The listing builds one solid part. Answer for the finished solid, in the listing's coordinates (mm). A direction names the side the tool comes from. Coordinates: 2 decimals unless noted, no trailing zeros. Order: outer loops, then holes, each group sorted by start corner. A loop starts at its lowest first (then second) coordinate and runs counter-clockwise, first axis right, second up. Notation, with made-up numbers: M -34.5,-28.75 L 22.5,-28.75 A21 cw 22.5,-6.75 Z; hole C -33.5,34.5 d7. An arc over 180 degrees is marked long. One line per item, written item: value. Start each with the question number.
Q1. This flat-tipped pin is pushed along its axis until it touches: pin 1 Ø2.5 at (y, z) = (-2, 4) entering from +X. Where does it stop, or does it pass through?
Q2. For faces 1 (the cylindrical face through (3, 4, 1)), 2 (the flat face through (-3, 0, 2.5)), determine the directions among +Z, -Z, +X, -X, +Y, -Y from which every point of the face is accessible in a straight line to the end or side of a thin tool.
Q3. The part is cut by section D-D on z = 8.25. Give the vertices of the cut face in (x, y), then the cut area to 3 significant figures.
Q4. The part is cut by section C-C on z = 5. Give the vertices of the cut face in (x, y).
Q5. The part is cut by section A-A on y = 0. Give the vertices of the cut face in (x, z), then the cut area to 3 significant figures.
Q6. Determine the mould class of faces 3 (the flat face through (-3, 0, 7.5)), 4 (the flat face through (-20, 0, 5)), 5 (the flat face through (-8, 0, 10)) for opening direction Z: pulls with the +Z half, pulls with the -Z half, needs draft (parallel to the pull), parting line crosses it, or undercut.
Q7. The part is cut by section B-B on x = -4.5. Give the vertices of the cut face in (y, z).
Q8. Straight lines are drawn through the part: line 1 along X through (y, z) = (0, 1.4); line 2 along Z through (x, y) = (-6, 0.25); line 3 along Y through (x, z) = (0, 8.15). For each, find the intervals that lie inside material, in ascending order. Write a range as [from, to].
```python
from build123d import *

# Parameters (mm, degrees)
CROQUIS1_W              = 25
CROQUIS1_H              = 10
CROQUIS1_R              = 1.5
SALIENTE_EXTRUIR1_DEPTH = 10
CROQUIS2_R              = 1.5
CORTAR_EXTRUIR1_DEPTH   = 14
CROQUIS3_W              = 5
CROQUIS3_H              = 10
CORTAR_EXTRUIR2_DEPTH   = 16.5
CUT_EXTRUDE1_DEPTH      = 10


with BuildPart() as part:
    # Croquis1 → Saliente-Extruir1 (new body)
    with BuildSketch(Plane.XY):
        with Locations((-7.5, 0)):
            Rectangle(CROQUIS1_W, CROQUIS1_H)
        Circle(CROQUIS1_R, mode=Mode.SUBTRACT)
    extrude(amount=SALIENTE_EXTRUIR1_DEPTH)

    # Croquis2 → Cortar-Extruir1 (cut)
    with BuildSketch(Plane(origin=(0, 5, 0), x_dir=(1, 0, 0), z_dir=(0, 1, 0))):
        with Locations(Location((-15, -5, 0), (0, 0, 180))):
            Circle(CROQUIS2_R)
    extrude(amount=-CORTAR_EXTRUIR1_DEPTH, mode=Mode.SUBTRACT)

    # Croquis3 → Cortar-Extruir2 (cut)
    with BuildSketch(Plane(origin=(5, 0, 0), x_dir=(0, 0, -1), z_dir=(1, 0, 0))):
        with Locations((-5, 0)):
            Rectangle(CROQUIS3_W, CROQUIS3_H)
    extrude(amount=-CORTAR_EXTRUIR2_DEPTH, mode=Mode.SUBTRACT)

    # Sketch1 → Cut-Extrude1 (cut)
    with BuildSketch(Plane.XY.offset(10)):
        with BuildLine():
            Line((0, 5), (5.992915048, 5))
            Line((5.992915048, 5), (5.992915048, -6.748814934))
            Line((5.992915048, -6.748814934), (0, -5))
            ThreePointArc((0, -5), (2.680080756, -4.221038633), (4.525089765, -2.126866856))
            Line((4.525089765, -2.126866856), (4.525089765, 2.126866856))
            ThreePointArc((4.525089765, 2.126866856), (2.680080756, 4.221038633), (0, 5))
        make_face()
    extrude(amount=-CUT_EXTRUDE1_DEPTH, mode=Mode.SUBTRACT)


solid = part.part
```
Output:
1. pin 1: stops at x = -11.5
2. face 1: +Z, -Z, +X, +Y
2. face 2: +X, +Y, -Y
3. outline: M -20,-5 L 0,-5 A5 ccw 4.53,-2.13 L 4.53,2.13 A5 ccw 0,5 L -20,5 Z; hole C 0,0 d3
3. area: 231 mm^2
4. outline: M -20,-5 L -16.5,-5 L -16.5,5 L -20,5 Z; M -13.5,-5 L -11.5,-5 L -11.5,5 L -13.5,5 Z
5. outline: M -20,0 L -1.5,0 L -1.5,2.5 L -11.5,2.5 L -11.5,7.5 L -1.5,7.5 L -1.5,10 L -20,10 Z; M 1.5,0 L 4.53,0 L 4.53,2.5 L 1.5,2.5 Z; M 1.5,7.5 L 4.53,7.5 L 4.53,10 L 1.5,10 Z; hole C -15,5 d3
5. area: 143 mm^2
6. face 3: undercut
6. face 4: needs draft
6. face 5: pulls with the +Z half
7. outline: M -5,0 L 5,0 L 5,2.5 L -5,2.5 Z; M -5,7.5 L 5,7.5 L 5,10 L -5,10 Z
8. line 1: x = [-20, -1.5], [1.5, 4.53]
8. line 2: z = [0, 2.5], [7.5, 10]
8. line 3: y = [-5, -1.5], [1.5, 5]
